from build123d import *

# Parameters (mm, degrees)
F0_R     = 41.071152
F1_DEPTH = 2
F3_DEPTH = 30


with BuildPart() as f1:
    # F0 (on Top) → F1 (new body)
    with BuildSketch(Plane.XY):
        Circle(F0_R)
    extrude(amount=F1_DEPTH)

    # F2 (on face) → F3 (join)
    with BuildSketch(Plane.XY.offset(2)):
        Polygon((40.473684, -6.980005), (-14.19198, 38.541241), (-26.281704, -31.561236), align=None)
    extrude(amount=F3_DEPTH)


solid = f1.part
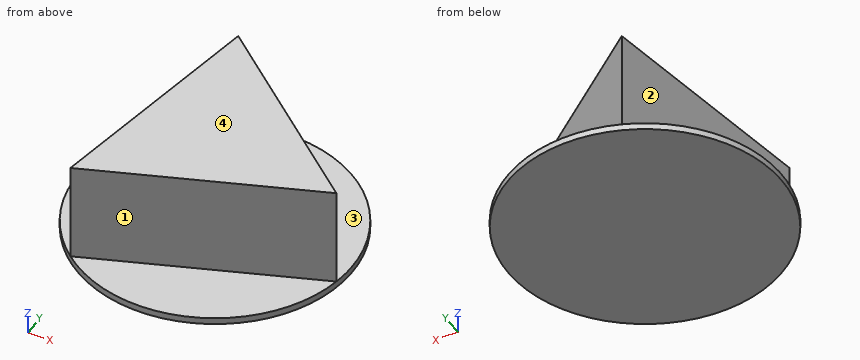
Check sheet for the modelled part. Datum: model origin and axes. Units: mm. Face numbers are marked on the shaded views. A direction names the side the tool comes from. Give positions to 0.01 mm unless a question says otherwise; leave off trailing zeros. Order: outer loops, then holes, each group sorted by start corner. A loop starts at its lowest first (then second) coordinate and runs counter-clockwise, first axis right, second up. Notation, with made-up numbers: M 44.25,88.5 L 70.25,88.5 A16 cw 70.25,109.5 Z; hole C 7,2.5 d10. An arc over 180 degrees is marked long. Answer as CSV lines item,"result". Start each with the question number.
Item 1: Gauge pin test, flat ends, axial feed: P1, Ø12, axis at x = 16.5, z = 13.5, coming from the +Y side; P2, Ø5, axis at x = 7.5, z = 29, coming from the +Y side; P3, Ø8, axis at x = -9.5, y = -30, coming from the +Z side. Record the tip position at first contact, or that the pin passes through.
Item 2: Thickness scan on line 1 (Z direction, x = 30, y = 15); line 2 (X direction, y = 2, z = 26); line 3 (Y direction, x = 27, z = 27). Record the ranges inside material, lowest first. Write a range as [from, to].
Item 3: Cross-section at C-C on z = 7. Enter the section's corners in (x, y), plus the area to 3 significant figures.
Item 4: Tool access check on the marked faces 1, 2, 3 and 4. Record the directions out of +Z, -Z, +X, -X, +Y, -Y that give a thin tool (end or side, any length) a straight path to the whole face; none if there is none.
Item 5: Cross-section at B-B on y = -2. Enter the section's corners in (x, z).
Item 6: Cross-section at A-A on x = -0.5. Enter the section's corners in (y, z).
Established:
1,P1,"stops at y = 17.98"
1,P2,"stops at y = 22.56"
1,P3,"stops at z = 2"
2,line 1,"z = [0, 2]"
2,line 2,"x = [-20.49, 29.69]"
2,line 3,"y = [-11.94, 4.24]"
3,outline,"M -26.28,-31.56 L 40.47,-6.98 L -14.19,38.54 Z"
3,area,"2,190 mm^2"
4,face 1,"+Z, +X, -Y"
4,face 2,"+Z, -X, +Y"
4,face 3,"+Z, +X, +Y"
4,face 4,"+Z, +X, -X, +Y, -Y"
5,outline,"M -41.02,0 L 41.02,0 L 41.02,2 L 34.49,2 L 34.49,32 L -21.18,32 L -21.18,2 L -41.02,2 Z"
6,outline,"M -41.07,0 L 41.07,0 L 41.07,2 L 27.14,2 L 27.14,32 L -22.07,32 L -22.07,2 L -41.07,2 Z"
